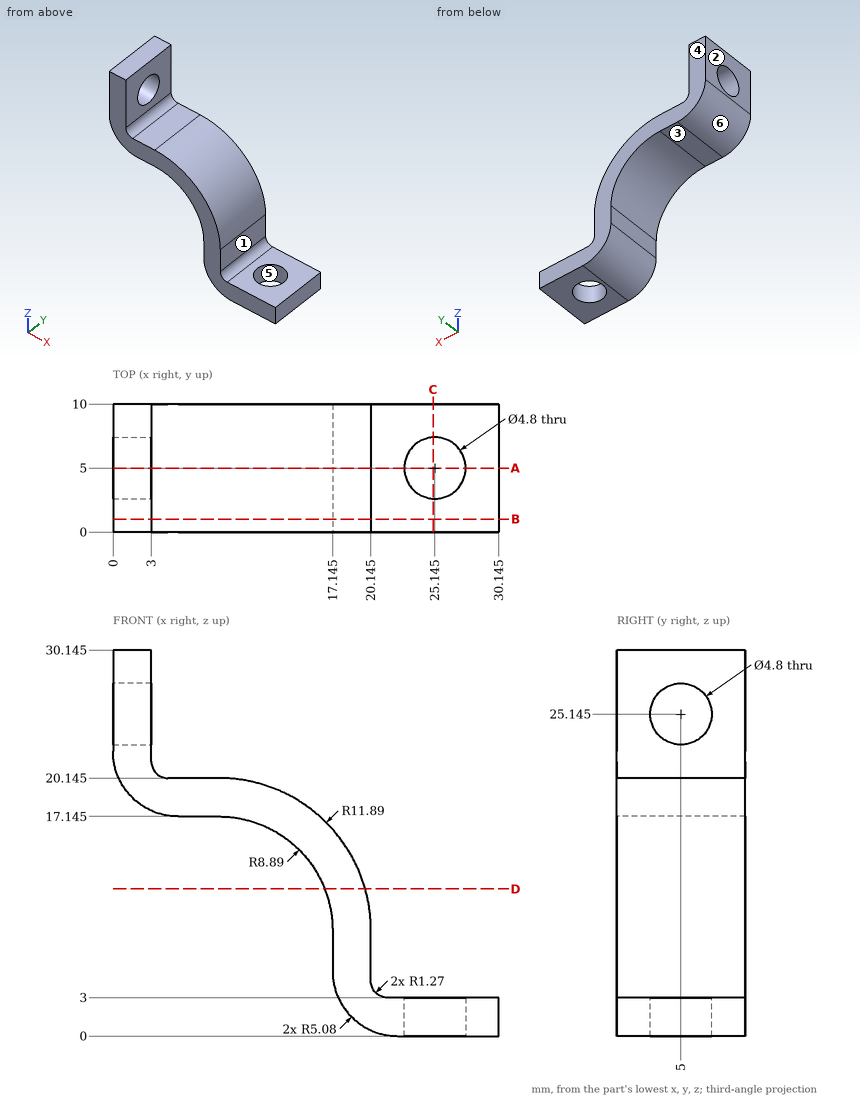
Part print with two shaded views. Sizes in mm from the minimum x, y, z corner. A direction names the side the tool comes from. Round coordinates to 2 decimals unless told otherwise and drop trailing zeros. Order: outer loops, then holes, each group sorted by start corner. A loop starts at its lowest first (then second) coordinate and runs counter-clockwise, first axis right, second up. Notation, with made-up numbers: (79, 69) -> (91, 69) arc R8 cw to (91, 76) -> close; hole circle Ø3 at (19, 13). An arc over 180 degrees is marked (long way). One line per question, with ' | ' between items.
Q1. Slice it at D-D (z = 11.5). Write the cut outline in (x, y), then the cut area to 3 significant figures.
Completed:
outline: (16.53, 0) -> (19.69, 0) -> (19.69, 10) -> (16.53, 10) -> close | area: 31.6 mm^2
Q2. Drop flat-ended pins along their axis: pin 1 (2 mm diameter, centred on x = 6.5, y = 3.5, fed in from +Z) (3 decimals); pin 2 (5 mm diameter, centred on y = 4.5, z = 23.5, fed in from +X); pin 3 (2 mm diameter, centred on x = 17, y = 4.5, fed in from +Z); pin 4 (4.5 mm diameter, centred on y = 5, z = 25.145, fed in from +X) (3 decimals). Give the stop position or say it passes through.
Completed:
pin 1: stops at z = 20.145 | pin 2: stops at x = 3.07 | pin 3: stops at z = 17.28 | pin 4: passes through
Q3. Slice it at B-B (y = 1). Write the cut outline in (x, z) (3 decimals).
Completed:
outline: (0, 22.225) arc R5.08 ccw to (5.08, 17.145) -> (8.255, 17.145) arc R8.89 cw to (17.145, 8.255) -> (17.145, 5.08) arc R5.08 ccw to (22.225, 0) -> (30.145, 0) -> (30.145, 3) -> (21.415, 3) arc R1.27 cw to (20.145, 4.27) -> (20.145, 8.255) arc R11.89 ccw to (8.255, 20.145) -> (4.27, 20.145) arc R1.27 cw to (3, 21.415) -> (3, 30.145) -> (0, 30.145) -> close
Q4. Probe probe 1 along X at (y, z) = (2.25, 6) (3 decimals); probe 2 along X at (y, z) = (7, 22.5); probe 3 along Y at (x, z) = (26.5, 2). List the from-to ranges inside material, lowest first.
Completed:
probe 1: x = 17.145 to 20.145 | probe 2: x = 0 to 3 | probe 3: y = 0 to 3.02, 6.98 to 10
Q5. Which spindle directions (+Z, -Z, +X, -X, +Y, -Y) get a long thin tool onto all of the face, cutting with end or side? Do the marked faces 1, 2 and 3. Say none if no direction does.
Completed:
face 1: +Z, +X, +Y, -Y | face 2: +Z, -Z, -X, +Y, -Y | face 3: -Z, -X, +Y, -Y
Q6. Slice it at C-C (x = 25). Write the cut outline in (y, z), then the cut area to 3 significant figures.
Completed:
outline: (0, 0) -> (2.6, 0) -> (2.6, 3) -> (0, 3) -> close; (7.4, 0) -> (10, 0) -> (10, 3) -> (7.4, 3) -> close | area: 15.6 mm^2
Q7. Slice it at A-A (y = 5). Write the cut outline in (x, z) (3 decimals).
Completed:
outline: (0, 22.225) arc R5.08 ccw to (5.08, 17.145) -> (8.255, 17.145) arc R8.89 cw to (17.145, 8.255) -> (17.145, 5.08) arc R5.08 ccw to (22.225, 0) -> (22.745, 0) -> (22.745, 3) -> (21.415, 3) arc R1.27 cw to (20.145, 4.27) -> (20.145, 8.255) arc R11.89 ccw to (8.255, 20.145) -> (4.27, 20.145) arc R1.27 cw to (3, 21.415) -> (3, 22.745) -> (0, 22.745) -> close; (0, 27.545) -> (3, 27.545) -> (3, 30.145) -> (0, 30.145) -> close; (27.545, 0) -> (30.145, 0) -> (30.145, 3) -> (27.545, 3) -> close
Q8. Two-plate mould, pull along X, no slides. Class the marked faces 4, 5 and 6: released by +X, released by -X, zero draft, split by the parting line, or undercut.
Completed:
face 4: zero draft | face 5: undercut | face 6: released by -X
